Answer from the drawing. Dimensions are ordinates in mm from the lowest x, y and z of the part. A direction names the side the tool comes from. Coordinates: 2 decimals unless noted, no trailing zeros. Loops run counter-clockwise (first coordinate to the right, second up) from the corner with the lowest first, then second, coordinate; pieces in that order, holes last.
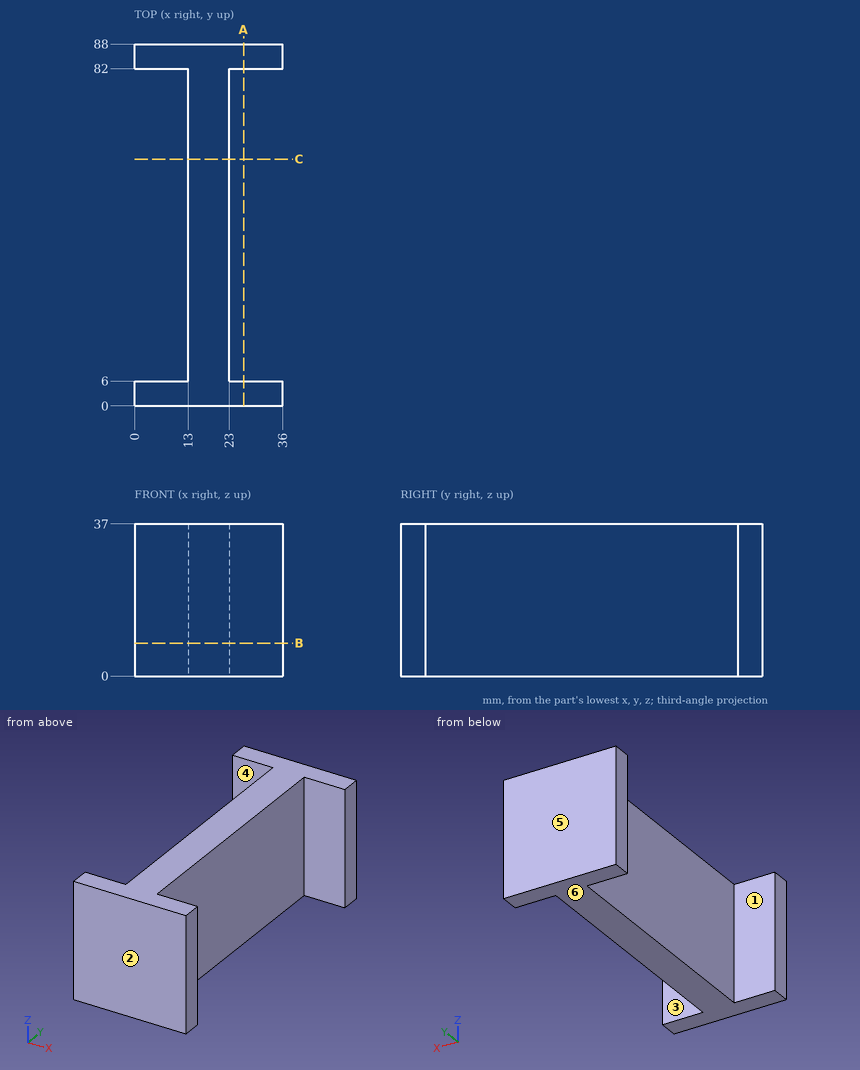
Item 1: Which of the six approach directions +Z, -Z, +X, -X, +Y, -Y give full straight-line access (tool end or side, diameter ignored) to the marked faces 1, 2 and 3?
Numbers:
face 1: +Z, -Z, -X
face 2: +Z, -Z, +X, -X, -Y
face 3: +Z, -Z, +X
Item 2: A cutting plane is placed at C-C on y = 60. Determine the outline of the cut face in (x, z), then the cut area to 3 significant figures.
Numbers:
outline: (13, 0) - (23, 0) - (23, 37) - (13, 37) - close
area: 370 mm2
Item 3: Find the intervals of material crossed by line 1 along Y through (x, z) = (32, 21); line 2 along X through (y, z) = (38, 4.5), in increasing order.
Numbers:
line 1: y = 0 to 6, 82 to 88
line 2: x = 13 to 23
Item 4: A cutting plane is placed at A-A on x = 26.5. Determine the outline of the cut face in (y, z).
Numbers:
outline: (0, 0) - (6, 0) - (6, 37) - (0, 37) - close; (82, 0) - (88, 0) - (88, 37) - (82, 37) - close
Item 5: Given pin 1 (11 mm diameter, centred on y = 38.5, z = 25.5, fed in from -X); pin 2 (12 mm diameter, centred on x = 8.5, z = 27.5, fed in from -Y); pin 3 (3 mm diameter, centred on y = 77, z = 31.5, fed in from +X), each flat-ended and moving along its own axis, determine where each tip first touches the part or whether it passes through.
Numbers:
pin 1: stops at x = 13
pin 2: stops at y = 0
pin 3: stops at x = 23
Item 6: Determine the mould class of the marked faces 4, 5 and 6 for opening direction Y: released by +Y, released by -Y, zero draft, split by the parting line, or undercut.
Numbers:
face 4: undercut
face 5: released by +Y
face 6: zero draft
Item 7: A cutting plane is placed at B-B on z = 8. Determine the outline of the cut face in (x, y).
Numbers:
outline: (0, 0) - (36, 0) - (36, 6) - (23, 6) - (23, 82) - (36, 82) - (36, 88) - (0, 88) - (0, 82) - (13, 82) - (13, 6) - (0, 6) - close
